Here's the drawing with two shaded views (mm, measured from the low corner). I have some questions. Give positions to 0.01 mm unless a question says otherwise; leave off trailing zeros. Loops run counter-clockwise (first coordinate to the right, second up) from the corner with the lowest first, then second, coordinate; pieces in that order, holes last.
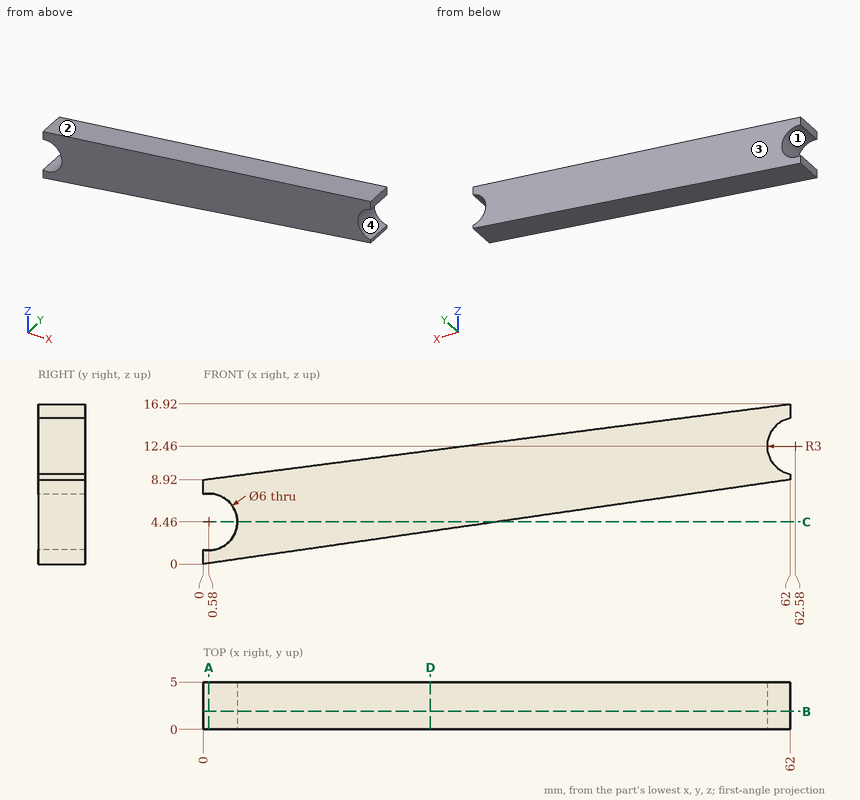
(1) Thinking about a two-plate mould opening in X: for the marked faces 1, 2, 3 and 4, which applies, pulls with the +X half, pulls with the -X half, needs draft (parallel to the pull), parting line crosses it, or undercut?
Returned:
face 1: undercut
face 2: pulls with the -X half
face 3: needs draft
face 4: pulls with the +X half
(2) Suppose I cut it at D-D on x = 24. List the corners of the cut face in (y, z) for me.
Returned:
outline: (0, 3.45) - (5, 3.45) - (5, 12.02) - (0, 12.02) - close
(3) Suppose I cut it at A-A on x = 0.58. List the corners of the cut face in (y, z) for me, plus the area to 3 significant figures.
Returned:
outline: (0, 0.08) - (5, 0.08) - (5, 1.46) - (0, 1.46) - close; (0, 7.46) - (5, 7.46) - (5, 8.99) - (0, 8.99) - close
area: 14.6 mm2
(4) Please list where these lines run through material, in increasing order: probe 1 along Z at (x, y) = (0.58, 3); probe 2 along Z at (x, y) = (53, 2.2); probe 3 along Z at (x, y) = (55, 3.35).
Returned:
probe 1: z = 0.08 to 1.46, 7.46 to 8.99
probe 2: z = 7.63 to 15.76
probe 3: z = 7.91 to 16.02
(5) Suppose I cut it at C-C on z = 4.46. List the corners of the cut face in (x, y) for me, plus the area to 3 significant figures.
Returned:
outline: (3.58, 0) - (31, 0) - (31, 5) - (3.58, 5) - close
area: 137 mm2
(6) Will this pin go through, and if not, where does the flat tip stop? P1, Ø3, axis at x = 55.5, y = 0.5, coming from the -Z side.
Returned:
P1: stops at z = 7.77
(7) Suppose I cut it at B-B on y = 1.9. List the corners of the cut face in (x, z) for me.
Returned:
outline: (0, 0) - (62, 8.92) - (62, 9.52) arc R3 cw to (62, 15.4) - (62, 16.92) - (0, 8.92) - (0, 7.4) arc R3 cw (long way) to (0, 1.52) - close
